```python
from build123d import *

# Parameters (mm, degrees)
BOX006_W     = 185
BOX006_H     = 185
BOX006_DEPTH = 8
BOX005_W     = 200
BOX005_H     = 200
BOX005_DEPTH = 5


with BuildPart() as cube006:
    # Box006 → Box006 (new body)
    with BuildSketch(Plane(origin=(7.5, 7.5, 93), x_dir=(1, 0, 0), z_dir=(0, 0, 1))):
        with Locations((92.5, 92.5)):
            Rectangle(BOX006_W, BOX006_H)
    extrude(amount=BOX006_DEPTH)


with BuildPart() as lid:
    # Box005 → Box005 (new body)
    with BuildSketch(Plane.XY.offset(96)):
        with Locations((100, 100)):
            Rectangle(BOX005_W, BOX005_H)
    extrude(amount=BOX005_DEPTH)

    # Fusion002: union Cube006
    add(cube006.part)


solid = lid.part
```
Part model, mm, in its own coordinate system. Coordinates: 2 decimals unless noted, no trailing zeros. Write each loop counter-clockwise with the first axis right and the second up, starting at its lowest first coordinate (ties: lowest second). Pieces come first, ordered by that corner, then holes.
Item 1: Probe line 1 (X direction, y = 12.5, z = 94.25). List the from-to ranges inside material, lowest first.
Item 2: Slice it at A-A (y = 112). Write the cut outline in (x, z).
Item 3: Mould opens along Y. For faces 1 (the face through (99, 0, 98)), 2 (the face through (99, 200, 98)), 3 (the face through (92, 4, 96)) say: released by +Y, released by -Y, zero draft, split by the parting line, or undercut.
Item 4: Slice it at C-C (z = 94.5). Write the cut outline in (x, y), and give its area (3 significant figures).
Item 5: Pin check, flat tips, straight feed: pin 1 (1.5 mm diameter, centred on y = 111, z = 94.5, fed in from -X); pin 2 (0.9 mm diameter, centred on x = 70.5, z = 94.5, fed in from -Y); pin 3 (0.9 mm diameter, centred on x = 83.5, z = 94, fed in from +Y). Stop position of each tip, or through.
Results found:
1. line 1: x = 7.5 to 192.5
2. outline: (0, 96) - (7.5, 96) - (7.5, 93) - (192.5, 93) - (192.5, 96) - (200, 96) - (200, 101) - (0, 101) - close
3. face 1: released by -Y
3. face 2: released by +Y
3. face 3: zero draft
4. outline: (7.5, 7.5) - (192.5, 7.5) - (192.5, 192.5) - (7.5, 192.5) - close
4. area: 34,200 mm2
5. pin 1: stops at x = 7.5
5. pin 2: stops at y = 7.5
5. pin 3: stops at y = 192.5
